Source: CAD feature listing. Evaluate the final solid. Frame: model axes, mm. Face numbers are marked on the shaded views. Round coordinates to 2 decimals unless told otherwise and drop trailing zeros. Loops run counter-clockwise (first coordinate to the right, second up) from the corner with the lowest first, then second, coordinate; pieces in that order, holes last.
Item 1: Pull-direction query (X, two-part tool) for the marked faces 1, 2 and 3; classes: released by +X, released by -X, zero draft, split by the parting line, or undercut.
Item 2: Section query D-D on y = -1.25. Return loops of the section in (x, z), then the cut area to 3 significant figures.
Item 3: First-contact query: P1, Ø1.3, axis at x = 4, y = -20.5, coming from the -Z side. Flat tip, straight axial feed; report the tip coordinate or a pass-through.
Item 4: Section query C-C on z = 3.1. Return loops of the section in (x, y), then the cut area to 3 significant figures.
Item 5: Section query B-B on x = 1.75. Return loops of the section in (y, z).
Item 6: Section query A-A on y = -20.5. Return loops of the section in (x, z).
Item 7: Ray query, L1, parallel to Y at x = 4, z = 2.35; L2, parallel to X at y = -20.25, z = 1.8; L3, parallel to Y at x = 0, z = 1.05. Return the intervals inside material, ascending.
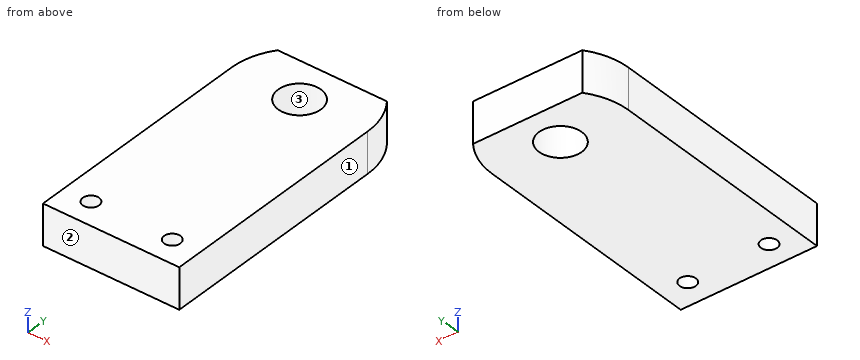
```python
from build123d import *

# Parameters (mm, degrees)
RESSALTO_EXTRUS_O1_DEPTH                = 4
FURO_ROSCADO_DE_M2X0_41_D               = 1.6
FURO_ROSCADO_PARA_CONDU_TE_DE_M4X0_71_D = 4.2


with BuildPart() as part:
    # Esboço1 → Ressalto-extrusão1 (new body)
    with BuildSketch(Plane.XY):
        with BuildLine():
            Line((-6.7, 0), (-6.7, -23))
            Line((-6.7, -23), (6.7, -23))
            Line((6.7, -23), (6.7, 0))
            ThreePointArc((6.7, 0), (6.360114404, 2.10688034), (5.37494186, 4))
            Line((5.37494186, 4), (-5.37494186, 4))
            ThreePointArc((-5.37494186, 4), (-6.360114404, 2.10688034), (-6.7, 0))
        make_face()
    extrude(amount=RESSALTO_EXTRUS_O1_DEPTH)

    # Furo roscado de M2x0.41 (through all)
    with Locations(Plane(origin=(-4, -20.5, 4), x_dir=(1, 0, 0), z_dir=(0, 0, 1))):
        with Locations((0, 0), (8, 0)):
            Hole(FURO_ROSCADO_DE_M2X0_41_D / 2)

    # Furo roscado para conduíte de M4x0.71 (through all)
    with Locations(Plane.XY.offset(4)):
        with Locations((0, 0)):
            Hole(FURO_ROSCADO_PARA_CONDU_TE_DE_M4X0_71_D / 2)


solid = part.part
```
Data:
1. face 1: released by +X
1. face 2: zero draft
1. face 3: undercut
2. outline: (-6.7, 0) - (-1.69, 0) - (-1.69, 4) - (-6.7, 4) - close; (1.69, 0) - (6.7, 0) - (6.7, 4) - (1.69, 4) - close
2. area: 40.1 mm2
3. P1: passes through
4. outline: (-6.7, -23) - (6.7, -23) - (6.7, 0) arc R6.7 ccw to (5.37, 4) - (-5.37, 4) arc R6.7 ccw to (-6.7, 0) - close; hole circle Ø1.6 at (-4, -20.5); hole circle Ø4.2 at (0, 0); hole circle Ø1.6 at (4, -20.5)
4. area: 341 mm2
5. outline: (-23, 0) - (-1.16, 0) - (-1.16, 4) - (-23, 4) - close; (1.16, 0) - (4, 0) - (4, 4) - (1.16, 4) - close
6. outline: (-6.7, 0) - (-4.8, 0) - (-4.8, 4) - (-6.7, 4) - close; (-3.2, 0) - (3.2, 0) - (3.2, 4) - (-3.2, 4) - close; (4.8, 0) - (6.7, 0) - (6.7, 4) - (4.8, 4) - close
7. L1: y = -23 to -21.3, -19.7 to 4
7. L2: x = -6.7 to -4.76, -3.24 to 3.24, 4.76 to 6.7
7. L3: y = -23 to -2.1, 2.1 to 4
